from build123d import *

# Parameters (mm, degrees)
SKETCH_1_W           = 140
SKETCH_1_H           = 320
EXTRUDE_1_DEPTH      = 5
SKETCH_2_R           = 46.5
SKETCH_2_R_2         = 37.5
SKETCH_2_R_3         = 2.1
CUT_EXTRUDE_1_DEPTH  = 5
CUT_EXTRUDE_2_DEPTH  = 5
SKETCH_4_R           = 2.15
CUT_EXTRUDE_3_DEPTH  = 5
SKETCH_5_R           = 2.1
CUT_EXTRUDE_4_DEPTH  = 15
CUT_EXTRUDE_5_DEPTH  = 10
SKETCH_7_R           = 1.6
CUT_EXTRUDE_6_DEPTH  = 327
FILLET_1_R           = 2
FILLET_2_R           = 2
SKETCH_9_R           = 2.6
CUT_EXTRUDE_8_DEPTH  = 10
SKETCH_10_R          = 2.6
CUT_EXTRUDE_9_DEPTH  = 10
SKETCH_11_R          = 2.6
CUT_EXTRUDE_10_DEPTH = 10
SKETCH_12_R          = 1.6
CUT_EXTRUDE_11_DEPTH = 10
SKETCH_13_R          = 2.1
CUT_EXTRUDE_12_DEPTH = 10
CUT_EXTRUDE_13_DEPTH = 10
FILLET_3_R           = 3
FILLET_5_R           = 3
FILLET_6_R           = 3
SKETCH_15_R          = 1.6
CUT_EXTRUDE_14_DEPTH = 10


with BuildPart() as part:
    # 草图1 → 凸台-拉伸1 (new body)
    with BuildSketch(Plane.XY):
        Rectangle(SKETCH_1_W, SKETCH_1_H)
    extrude(amount=EXTRUDE_1_DEPTH)

    # 草图2 → 切除-拉伸1 (cut)
    with BuildSketch(Plane.XY.offset(5)):
        with Locations((0, 75)):
            Circle(SKETCH_2_R)
        with Locations((0, -75)):
            Circle(SKETCH_2_R_2)
        with Locations((42.5, -75)):
            Circle(SKETCH_2_R_3)
        with Locations((30.0520382, -105.0520382)):
            Circle(SKETCH_2_R_3)
        with Locations((0, -117.5)):
            Circle(SKETCH_2_R_3)
        with Locations((-30.0520382, -105.0520382)):
            Circle(SKETCH_2_R_3)
        with Locations((-42.5, -75)):
            Circle(SKETCH_2_R_3)
        with Locations((-30.0520382, -44.9479618)):
            Circle(SKETCH_2_R_3)
        with Locations((0, -32.5)):
            Circle(SKETCH_2_R_3)
        with Locations((30.0520382, -44.9479618)):
            Circle(SKETCH_2_R_3)
    extrude(amount=-CUT_EXTRUDE_1_DEPTH, mode=Mode.SUBTRACT)

    # 草图3 → 切除-拉伸2 (cut)
    with BuildSketch(Plane.XY.offset(5)):
        Polygon((-43.553654222, -67.783407733), (-17.685027311, -78.49854384), (-10.031358664, -60.020953189), (-35.899985574, -49.305817083), align=None)
    extrude(amount=-CUT_EXTRUDE_2_DEPTH, mode=Mode.SUBTRACT)

    # 草图4 → 切除-拉伸3 (cut)
    with BuildSketch(Plane.XY.offset(5)):
        with Locations((0, -20)):
            Circle(SKETCH_4_R)
        with Locations((27.5, -27.368602792)):
            Circle(SKETCH_4_R)
        with Locations((47.631397208, -47.5)):
            Circle(SKETCH_4_R)
        with Locations((55, -75)):
            Circle(SKETCH_4_R)
        with Locations((47.631397208, -102.5)):
            Circle(SKETCH_4_R)
        with Locations((27.5, -122.631397208)):
            Circle(SKETCH_4_R)
        with Locations((0, -130)):
            Circle(SKETCH_4_R)
        with Locations((-27.5, -122.631397208)):
            Circle(SKETCH_4_R)
        with Locations((-47.631397208, -102.5)):
            Circle(SKETCH_4_R)
        with Locations((-55, -75)):
            Circle(SKETCH_4_R)
        with Locations((-47.631397208, -47.5)):
            Circle(SKETCH_4_R)
        with Locations((-27.5, -27.368602792)):
            Circle(SKETCH_4_R)
    extrude(amount=-CUT_EXTRUDE_3_DEPTH, mode=Mode.SUBTRACT)

    # 草图5 → 切除-拉伸4 (cut)
    with BuildSketch(Plane(origin=(0, 0, 0), x_dir=(-1, 0, 0), z_dir=(0, 0, -1))):
        with Locations((0, 130)):
            Circle(SKETCH_5_R)
        with Locations((27.5, 122.631397208)):
            Circle(SKETCH_5_R)
        with Locations((47.631397208, 102.5)):
            Circle(SKETCH_5_R)
        with Locations((55, 75)):
            Circle(SKETCH_5_R)
        with Locations((47.631397208, 47.5)):
            Circle(SKETCH_5_R)
        with Locations((27.5, 27.368602792)):
            Circle(SKETCH_5_R)
        with Locations((0, 20)):
            Circle(SKETCH_5_R)
        with Locations((-27.5, 27.368602792)):
            Circle(SKETCH_5_R)
        with Locations((-47.631397208, 47.5)):
            Circle(SKETCH_5_R)
        with Locations((-55, 75)):
            Circle(SKETCH_5_R)
        with Locations((-47.631397208, 102.5)):
            Circle(SKETCH_5_R)
        with Locations((-27.5, 122.631397208)):
            Circle(SKETCH_5_R)
    extrude(amount=-CUT_EXTRUDE_4_DEPTH, mode=Mode.SUBTRACT)

    # 草图6 → 切除-拉伸5 (cut)
    with BuildSketch(Plane.XY.offset(5)):
        Polygon((30, 160), (70, 120), (70, 160), align=None)
        Polygon((70, -120), (70, -160), (30, -160), align=None)
    extrude(amount=-CUT_EXTRUDE_5_DEPTH, mode=Mode.SUBTRACT)

    # 草图7 → 切除-拉伸6 (cut)
    with BuildSketch(Plane.XY.offset(5)):
        with Locations((41.715728753, -144.04163056)):
            Circle(SKETCH_7_R)
        with Locations((55.857864376, -129.899494937)):
            Circle(SKETCH_7_R)
        with Locations(Location((55.857864376, 129.899494937, 0), (0, 0, 180))):
            Circle(SKETCH_7_R)
        with Locations(Location((41.715728753, 144.04163056, 0), (0, 0, 180))):
            Circle(SKETCH_7_R)
    extrude(amount=-CUT_EXTRUDE_6_DEPTH, mode=Mode.SUBTRACT)

    # 圆角1
    fillet_1_edges = [part.edges().sort_by_distance(p)[0] for p in [
        (30, 160, 2.5),
        (70, 120, 2.5),
        (30, -160, 2.5),
        (70, -120, 2.5),
        (-37.217762979, -70.407819816, 2.5),
        (-29.564094332, -51.930229166, 2.5),
        (-35.899985574, -49.305817083, 2.5),
        (-70, -160, 2.5),
        (-70, 160, 2.5),
    ]]
    fillet(fillet_1_edges, radius=FILLET_1_R)

    # 圆角2
    fillet_2_edges = [part.edges().sort_by_distance(p)[0] for p in [
        (-43.553654222, -67.783407733, 2.5),
    ]]
    fillet(fillet_2_edges, radius=FILLET_2_R)

    # 草图9 → 切除-拉伸8 (cut)
    with BuildSketch(Plane.XY.offset(5)):
        with Locations((-23.7, 0)):
            Circle(SKETCH_9_R)
        with Locations((-23.7, -23.5)):
            Circle(SKETCH_9_R)
        with Locations((-23.7, -151)):
            Circle(SKETCH_9_R)
        with Locations((-23.7, -127.5)):
            Circle(SKETCH_9_R)
    extrude(amount=-CUT_EXTRUDE_8_DEPTH, mode=Mode.SUBTRACT)

    # 草图10 → 切除-拉伸9 (cut)
    with BuildSketch(Plane.XY.offset(5)):
        with Locations((-60, -143)):
            Circle(SKETCH_10_R)
        with Locations(Location((-60, 143, 0), (0, 0, 180))):
            Circle(SKETCH_10_R)
        with Locations((-42, 143)):
            Circle(SKETCH_10_R)
        with Locations(Location((-42, -143, 0), (0, 0, 180))):
            Circle(SKETCH_10_R)
    extrude(amount=-CUT_EXTRUDE_9_DEPTH, mode=Mode.SUBTRACT)

    # 草图11 → 切除-拉伸10 (cut)
    with BuildSketch(Plane.XY.offset(5)):
        with Locations((-23.7, 152)):
            Circle(SKETCH_11_R)
    extrude(amount=-CUT_EXTRUDE_10_DEPTH, mode=Mode.SUBTRACT)

    # 草图12 → 切除-拉伸11 (cut)
    with BuildSketch(Plane.XY.offset(5)):
        with Locations((67, -104.585786438)):
            Circle(SKETCH_12_R)
        with Locations((67, -84.585786438)):
            Circle(SKETCH_12_R)
        with Locations((67, 94.585786438)):
            Circle(SKETCH_12_R)
        with Locations((67, 74.585786438)):
            Circle(SKETCH_12_R)
        with Locations((67, 34.585786438)):
            Circle(SKETCH_12_R)
        with Locations((67, 14.585786438)):
            Circle(SKETCH_12_R)
    extrude(amount=-CUT_EXTRUDE_11_DEPTH, mode=Mode.SUBTRACT)

    # 草图13 → 切除-拉伸12 (cut)
    with BuildSketch(Plane.XY.offset(5)):
        with Locations((20.786796564, 148)):
            Circle(SKETCH_13_R)
        with Locations((31.393398282, 137.393398282)):
            Circle(SKETCH_13_R)
        with Locations(Location((31.393398282, -137.393398282, 0), (0, 0, 180))):
            Circle(SKETCH_13_R)
        with Locations(Location((20.786796564, -148, 0), (0, 0, 180))):
            Circle(SKETCH_13_R)
    extrude(amount=-CUT_EXTRUDE_12_DEPTH, mode=Mode.SUBTRACT)

    # 草图14 → 切除-拉伸13 (cut)
    with BuildSketch(Plane.XY.offset(5)):
        Polygon((13.082912069, 13.840088814), (13.082912069, -11.76243836), (60.305351078, 1.038825227), align=None)
        Polygon((62.808709291, -3.114473625), (28.807148392, -12.33176423), (62.808709291, -50.678279663), align=None)
        Polygon((45.805341988, 35.251376217), (22.206313522, 13.840088814), (62.808709291, 3.011971197), align=None)
        Polygon((-56.619486608, 32.209554881), (-56.619486608, -36.253803925), (-32.797397419, -18.962637445), (-32.797397419, 12.07513926), align=None)
    extrude(amount=-CUT_EXTRUDE_13_DEPTH, mode=Mode.SUBTRACT)

    # 圆角3
    fillet_3_edges = [part.edges().sort_by_distance(p)[0] for p in [
        (62.808709291, -3.114473625, 2.5),
        (62.808709291, -50.678279663, 2.5),
        (28.807148392, -12.33176423, 2.5),
        (13.082912069, 13.840088814, 2.5),
        (60.305351078, 1.038825227, 2.5),
        (13.082912069, -11.76243836, 2.5),
    ]]
    fillet(fillet_3_edges, radius=FILLET_3_R)

    # 圆角5
    fillet_5_edges = [part.edges().sort_by_distance(p)[0] for p in [
        (45.805341988, 35.251376217, 2.5),
        (62.808709291, 3.011971197, 2.5),
        (22.206313522, 13.840088814, 2.5),
    ]]
    fillet(fillet_5_edges, radius=FILLET_5_R)

    # 圆角6
    fillet_6_edges = [part.edges().sort_by_distance(p)[0] for p in [
        (-32.797397419, -18.962637445, 2.5),
        (-56.619486608, -36.253803925, 2.5),
        (-56.619486608, 32.209554881, 2.5),
        (-32.797397419, 12.07513926, 2.5),
    ]]
    fillet(fillet_6_edges, radius=FILLET_6_R)

    # 草图15 → 切除-拉伸14 (cut)
    with BuildSketch(Plane.XY.offset(5)):
        with Locations((-67, -125)):
            Circle(SKETCH_15_R)
        with Locations((-67, -105)):
            Circle(SKETCH_15_R)
        with Locations((-67, -35)):
            Circle(SKETCH_15_R)
        with Locations((-67, -55)):
            Circle(SKETCH_15_R)
        with Locations(Location((-67, 55, 0), (0, 0, 180))):
            Circle(SKETCH_15_R)
        with Locations(Location((-67, 35, 0), (0, 0, 180))):
            Circle(SKETCH_15_R)
        with Locations(Location((-67, 105, 0), (0, 0, 180))):
            Circle(SKETCH_15_R)
        with Locations(Location((-67, 125, 0), (0, 0, 180))):
            Circle(SKETCH_15_R)
    extrude(amount=-CUT_EXTRUDE_14_DEPTH, mode=Mode.SUBTRACT)


solid = part.part
Source: CAD feature listing. Evaluate the final solid. Frame: model axes, mm. A direction names the side the tool comes from. Give positions to 0.01 mm unless a question says otherwise; leave off trailing zeros. Write each loop counter-clockwise with the first axis right and the second up, starting at its lowest first coordinate (ties: lowest second). Pieces come first, ordered by that corner, then holes. Notation, with made-up numbers: M 5.5,53 L 62.5,53 A19 ccw 62.5,71 Z; hole C -25.75,5 d7. An arc over 180 degrees is marked long. Return JSON: item names as keys, results as strings. Group by question number.
1) Cut plane C-C, the plane z = 3.55. Give the number of separate pieces and of enclosed holes in the cut face, plus the area to 3 significant figures.
2) Cut plane A-A, the plane y = 85.5. Output: boundary loops of the cut face in (x, z), plus the area to 3 significant figures.
3) Material intervals for line 1 along Y through (x, z) = (10, 1.45); line 2 along X through (y, z) = (-125.5, 1.55); line 3 along X through (y, z) = (-34, 1.5), sorted ascending. Write a range as [from, to].
4) Set-up query: faces 5 (the face through (53.694, 20.294, 2.535)), 6 (the face through (-1, 2, 0)). Return all of +Z, -Z, +X, -X, +Y, -Y with unobstructed straight access to the full face (end or side cutting, diameter ignored); none if empty.
5) Pull-direction query (Y, two-part tool) for faces 1 (the face through (50, 140, 3)), 2 (the face through (44.612, -30.156, 2.535)), 3 (the face through (50, -140, 3)), 4 (the face through (-1, 2, 5)); classes: pulls with the +Y half, pulls with the -Y half, needs draft (parallel to the pull), parting line crosses it, or undercut.
6) Cut plane B-B, the plane x = -11. Output: boundary loops of the cut face in (y, z), plus the area to 3 significant figures.
Recorded:
{
 "1": {"separate pieces": "1", "enclosed holes": "69", "area": "28,000 mm²"},
 "2": {"outline": "M -70,0 L -45.3,0 L -45.3,5 L -70,5 Z; M 45.3,0 L 70,0 L 70,5 L 45.3,5 Z", "area": "247 mm²"},
 "3": {"line 1": "y = [-160, -111.14], [-38.86, 29.59], [120.41, 160]", "line 2": "x = [-70, -68.52], [-65.48, -25.36], [-22.04, 64.5]", "line 3": "x = [-70, -68.25], [-65.75, -1.47], [1.47, 48.02], [62.81, 70]"},
 "4": {"face 5": "+Z, -Z", "face 6": "-Z, +X, -X, +Y, -Y"},
 "5": {"face 1": "pulls with the +Y half", "face 2": "undercut", "face 3": "pulls with the -Y half", "face 4": "needs draft"},
 "6": {"outline": "M -160,0 L -110.85,0 L -110.85,5 L -160,5 Z; M -39.15,0 L 29.82,0 L 29.82,5 L -39.15,5 Z; M 120.18,0 L 160,0 L 160,5 L 120.18,5 Z", "area": "790 mm²"}
}
